Can you work these out from the model? Positions are in its coordinate system, mm. A direction names the side the tool comes from. Coordinates: 2 decimals unless noted, no trailing zeros. Loops run counter-clockwise (first coordinate to the right, second up) from the corner with the lowest first, then second, coordinate; pieces in that order, holes last. Notation, with made-up numbers: (-29.5, -29) - (14.5, -29) arc R16 cw to (14.5, -3) - close; hole circle Ø9 at (10, 44.25). An arc over 180 degrees is marked (long way). Put each result on its own line as item: value. Start each with the question number.
from build123d import *

# Parameters (mm, degrees)
BOX033_W               = 5
BOX033_H               = 49
BOX033_DEPTH           = 74
BOX033_PITCH_ANGLE     = 29
PAD001_DEPTH           = 4
PAD_DEPTH              = 4
EXTRUDE044_DEPTH       = 6
EXTRUDE044_PITCH_ANGLE = -13
BOX032_W               = 47
BOX032_H               = 35
BOX032_DEPTH           = 12
BOX021_W               = 10
BOX021_H               = 3
BOX021_DEPTH           = 49
BOX021_PLACEMENT_ANGLE = 30
BOX020_W               = 5
BOX020_H               = 21.5
BOX020_DEPTH           = 52
BOX020_PITCH_ANGLE     = 29
CUT035_PLACEMENT_ANGLE = 70


with BuildPart() as obj1:
    # Box033 → Box033 (new body)
    with BuildSketch(Plane.XY):
        with Locations((2.5, 24.5)):
            Rectangle(BOX033_W, BOX033_H)
    extrude(amount=BOX033_DEPTH)


with BuildPart() as obj1_1:
    # Box033 pitch: moved
    add(obj1.part.rotate(Axis((0, 0, 0), (0, 1, 0)), BOX033_PITCH_ANGLE))


with BuildPart() as obj1_2:
    # Box033 placement: moved
    add(obj1_1.part.moved(Location((-34, -29, 0))))


with BuildPart() as pad001:
    # Sketch021 → Pad001 (new body)
    with BuildSketch(Plane.XY.offset(3)):
        with BuildLine():
            Line((-23.358564, -3.63874), (-23.358564, 3.63874))
            ThreePointArc((-6.004676, 24.074331), (-18.054345, 16.720651), (-23.358564, 3.63874))
            Line((-6.004676, 24.074331), (36.3059, 34.679668))
            ThreePointArc((36.87983, 32.765973), (37.506884, 33.996941), (36.3059, 34.679668))
            Line((36.87983, 32.765973), (-4.412486, 18.291349))
            ThreePointArc((-4.412486, 18.291349), (-14.077658, 11.396909), (-17.779108, 0.116478))
            Line((-17.779108, 0.116478), (-17.779108, -0.174905))
            ThreePointArc((-17.779108, -0.174905), (-14.075788, -11.431815), (-4.412486, -18.291349))
            Line((-4.412486, -18.291349), (36.879838, -32.765976))
            ThreePointArc((36.3059, -34.679668), (37.506883, -33.996945), (36.879838, -32.765976))
            Line((36.3059, -34.679668), (-6.004676, -24.074331))
            ThreePointArc((-23.358564, -3.63874), (-18.054345, -16.720651), (-6.004676, -24.074331))
        make_face()
    extrude(amount=PAD001_DEPTH)


with BuildPart() as pad:
    # Sketch020 → Pad (new body)
    with BuildSketch(Plane.XY):
        with BuildLine():
            Line((-28.053126, -17.5), (-28.053126, 17.5))
            Line((-28.053126, 17.5), (-11.404976, 29.852464))
            Line((-11.404976, 29.852464), (35.190344, 38.097016))
            ThreePointArc((37.911252, 29.600454), (40.755985, 35.195389), (35.190344, 38.097016))
            Line((37.911252, 29.600454), (-1.109137, 16.664622))
            ThreePointArc((-1.109137, 16.664622), (-9.755072, 10.323805), (-13.053126, 0.121796))
            Line((-13.053126, 0.121796), (-13.053126, -0.121796))
            ThreePointArc((-13.053126, -0.121796), (-9.755072, -10.323805), (-1.109137, -16.664622))
            Line((-1.109137, -16.664622), (37.911252, -29.600454))
            ThreePointArc((35.190344, -38.097016), (40.755985, -35.195389), (37.911252, -29.600454))
            Line((35.190344, -38.097016), (-11.404976, -29.852464))
            Line((-28.053126, -17.5), (-11.404976, -29.852464))
        make_face()
    extrude(amount=PAD_DEPTH)


with BuildPart() as extrude044:
    # Sketch016 → Extrude044 (new body)
    with BuildSketch(Plane.XY):
        Polygon((23.917763, 0), (13.167763, 10.75), (-16.832237, 10.75), (-16.832237, -10.75), (13.167763, -10.75), align=None)
    extrude(amount=EXTRUDE044_DEPTH)


with BuildPart() as extrude044_1:
    # Extrude044 pitch: moved
    add(extrude044.part.rotate(Axis((0, 0, 0), (0, 1, 0)), EXTRUDE044_PITCH_ANGLE))


with BuildPart() as extrude044_2:
    # Extrude044 placement: moved
    add(extrude044_1.part.moved(Location((10, -1.25, 41))))


with BuildPart() as obj2:
    # Box032 → Box032 (new body)
    with BuildSketch(Plane(origin=(-20, -15, 43), x_dir=(1, 0, 0), z_dir=(0, 0, 1))):
        with Locations((23.5, 17.5)):
            Rectangle(BOX032_W, BOX032_H)
    extrude(amount=BOX032_DEPTH)


with BuildPart() as obj3:
    # Box021 → Box021 (new body)
    with BuildSketch(Plane.XY):
        with Locations((5, 1.5)):
            Rectangle(BOX021_W, BOX021_H)
    extrude(amount=BOX021_DEPTH)


with BuildPart() as obj3_1:
    # Box021 placement: moved
    add(obj3.part.moved(Location((-26, -1, 6))).rotate(Axis((-26, -1, 6), (0, 1, 0)), BOX021_PLACEMENT_ANGLE))


with BuildPart() as stand:
    # Box020 → Box020 (new body)
    with BuildSketch(Plane.XY):
        with Locations((2.5, 10.75)):
            Rectangle(BOX020_W, BOX020_H)
    extrude(amount=BOX020_DEPTH)


with BuildPart() as stand_1:
    # Box020 pitch: moved
    add(stand.part.rotate(Axis((0, 0, 0), (0, 1, 0)), BOX020_PITCH_ANGLE))


with BuildPart() as stand_2:
    # Box020 placement: moved
    add(stand_1.part.moved(Location((-28, -11, 4))))

    # Fusion021: union obj3
    add(obj3_1.part)

    # Cut029: cut obj2
    add(obj2.part, mode=Mode.SUBTRACT)


with BuildPart() as stand_3:
    # Cut029 placement: moved
    add(stand_2.part.moved(Location((0, -1, 0))))

    # Fusion032: union Pad001, Pad, Extrude044
    add(pad001.part)
    add(pad.part)
    add(extrude044_2.part)

    # Cut035: cut obj1
    add(obj1_2.part, mode=Mode.SUBTRACT)


with BuildPart() as stand_4:
    # Cut035 placement: moved
    add(stand_3.part.moved(Location((86, 0, 16))).rotate(Axis((86, 0, 16), (0, -1, 0)), CUT035_PLACEMENT_ANGLE))


solid = stand_4.part
Q1. Will these pins go through, and if not, where does the flat tip stop? pin 1 (4 mm diameter, centred on x = 84.5, z = 23, fed in from -Y); pin 2 (25 mm diameter, centred on x = 54.5, z = 27.5, fed in from +Y); pin 3 (8.5 mm diameter, centred on x = 67.5, z = 18, fed in from +Y); pin 4 (3 mm diameter, centred on x = 54.5, y = -15, fed in from -Z).
Q2. I want a section at C-C on y = 7. List the corners of the cut face in (x, z) for me.
Q3. We'd pull the mould along Z, two halves only. Please class faces 5 (the flat face through (80.505, 0.536, 0.903)), 6 (the flat face through (86.305, -25.427, 32.857)), 7 (the flat face through (85.93, 29.3, 31.83)): released by +Z, released by -Z, zero draft, split by the parting line, or undercut.
Q4. I want a section at A-A on z = 46. List the corners of the cut face in (x, y) for me, and give its area (3 significant figures).
Q5. I want a section at B-B on x = 69.5. List the corners of the cut face in (y, z) for me.
Q6. I want a section at D-D on z = 59. List the corners of the cut face in (x, y) for me, and give its area (3 significant figures).
Q7. On a 3-axis mill with a long thin cutter (end or side, diameter ignored), from which of +Z, -Z, +X, -X, +Y, -Y can I reach the whole of each face in a straight line? I mean faces 1 (the flat face through (60.949, -7.07, 12.155)), 2 (the flat face through (86.13, -29.45, 32.39)), 3 (the cylindrical face through (76.2, -12.03, 5.08)), 4 (the flat face through (90.347, -23.042, 33.709)). Say none if no direction works.
Q8. Please list where these lines run through material, in increasing order: line 1 along Y through (x, z) = (63, 9); line 2 along Y through (x, z) = (56, 24); line 3 along Y through (x, z) = (94.5, 46). Write a range as [from, to].
Calculated:
1. pin 1: y = -33.3
1. pin 2: y = 9.5
1. pin 3: y = 1
1. pin 4: through
2. outline: (43.36, 27.34) - (76.02, -10.22) - (76.41, -10.36) - (82.02, 5.06) - (78.26, 6.43) - (76.6, 1.87) - (73.78, 2.9) - (72.37, -0.98) - (49.2, 25.67) - (52.8, 54.97) - (46.85, 55.7) - close
3. face 5: released by -Z
3. face 6: released by +Z
3. face 7: undercut
4. outline: (45.66, -12) - (51.7, -12) - (51.7, 9.5) - (45.66, 9.5) - close; (89.47, -32.94) - (92.66, -33.22) - (92.66, -37.26) - (96.92, -37.52) - (96.92, -27.62) - (92.66, -27.13) - (92.66, -30.52) - (89.47, -30.14) - close; (89.47, 30.14) - (92.66, 30.52) - (92.66, 27.13) - (96.92, 27.62) - (96.92, 37.52) - (92.66, 37.26) - (92.66, 33.22) - (89.47, 32.94) - close
4. area: 233 mm2
5. outline: (-12, -2.72) - (9.5, -2.72) - (9.5, 2.32) - (1, 2.32) - (1, 11.52) - (-2, 11.52) - (-2, 2.32) - (-12, 2.32) - close
6. outline: (47.25, -6.18) - (53.3, -5.44) - (53.3, 2.94) - (47.25, 3.68) - close
6. area: 55.1 mm2
7. face 1: -Y
7. face 2: -X, -Y
7. face 3: +Z
7. face 4: +Z, +X
8. line 1: [-12, 9.5]
8. line 2: [-2, 1]
8. line 3: [-37.37, -27.34], [27.34, 37.37]
